from build123d import *

# Parameters (mm, degrees)
SKETCH1_W           = 152.4
SKETCH1_H           = 152.4
BOSS_EXTRUDE1_DEPTH = 101.6
SHELL1_T            = -12.7
SKETCH2_R           = 5.08
CUT_EXTRUDE1_DEPTH  = 189.799073091


with BuildPart() as part:
    # Sketch1 → Boss-Extrude1 (new body)
    with BuildSketch(Plane(origin=(0, 0, 0), x_dir=(1, 0, 0), z_dir=(0, 1, 0))):
        Rectangle(SKETCH1_W, SKETCH1_H)
    extrude(amount=BOSS_EXTRUDE1_DEPTH)

    # Shell1
    shell1_openings = [part.faces().sort_by_distance(p)[0] for p in [
        (0, 101.6, 0),
    ]]
    offset(amount=SHELL1_T, openings=shell1_openings, kind=Kind.INTERSECTION)

    # Sketch2 → Cut-Extrude1 (cut, through all)
    with BuildSketch(Plane.XY.offset(-63.5)):
        with Locations(Location((-53.34, 22.86, 0), (0, 0, 180))):
            Circle(SKETCH2_R)
        with Locations(Location((53.34, 22.86, 0), (0, 0, 180))):
            Circle(SKETCH2_R)
    cut_extrude1 = extrude(amount=CUT_EXTRUDE1_DEPTH, mode=Mode.SUBTRACT)

    # Mirror1: Cut-Extrude1 across plane
    add(cut_extrude1.mirror(Plane.XY), mode=Mode.SUBTRACT)


solid = part.part
The listing builds one solid part. Answer for the finished solid, in the listing's coordinates (mm). A direction names the side the tool comes from. Give positions to 0.01 mm unless a question says otherwise; leave off trailing zeros. Write each loop counter-clockwise with the first axis right and the second up, starting at its lowest first coordinate (ties: lowest second). Pieces come first, ordered by that corner, then holes. Notation, with made-up numbers: (88, 14) - (119, 14) arc R17 ccw to (119, 26) - close; hole circle Ø3 at (61, -8.5). An arc over 180 degrees is marked (long way). Use a Markdown table: item, result.
1. Section B-B on y = 22.86 is taken. Write down the section's boundary in (x, z), plus the area to 3 significant figures.
Values follow:
| item | result |
|---|---|
| outline | (-76.2, -76.2) - (-58.42, -76.2) - (-58.42, -63.5) - (-63.5, -63.5) - (-63.5, 63.5) - (-58.42, 63.5) - (-58.42, 76.2) - (-76.2, 76.2) - close; (-48.26, -76.2) - (48.26, -76.2) - (48.26, -63.5) - (-48.26, -63.5) - close; (-48.26, 63.5) - (48.26, 63.5) - (48.26, 76.2) - (-48.26, 76.2) - close; (58.42, -76.2) - (76.2, -76.2) - (76.2, 76.2) - (58.42, 76.2) - (58.42, 63.5) - (63.5, 63.5) - (63.5, -63.5) - (58.42, -63.5) - close |
| area | 6,580 mm² |
2. Section A-A on x = -53.34 is taken. Write down the section's boundary in (y, z).
Values follow:
| item | result |
|---|---|
| outline | (0, -76.2) - (17.78, -76.2) - (17.78, -63.5) - (12.7, -63.5) - (12.7, 63.5) - (17.78, 63.5) - (17.78, 76.2) - (0, 76.2) - close; (27.94, -76.2) - (101.6, -76.2) - (101.6, -63.5) - (27.94, -63.5) - close; (27.94, 63.5) - (101.6, 63.5) - (101.6, 76.2) - (27.94, 76.2) - close |
3. Each of these flat-tipped pins is pushed along its axis until it touches: P1, Ø2, axis at x = -2.5, z = 56, coming from the -Y side; P2, Ø6, axis at x = 7.5, z = 32.5, coming from the +Y side. Where does it stop, or does it pass through?
Values follow:
| item | result |
|---|---|
| P1 | stops at y = 0 |
| P2 | stops at y = 12.7 |
4. Find the intervals of material crossed by probe 1 along X at (y, z) = (22.86, -68.5); probe 2 along X at (y, z) = (87.5, -28), in increasing order. Write a range as from..to.
Values follow:
| item | result |
|---|---|
| probe 1 | x = -76.2..-58.42, -48.26..48.26, 58.42..76.2 |
| probe 2 | x = -76.2..-63.5, 63.5..76.2 |
5. For a pull along Y with two mould halves and no side action, classify faces 3 (the flat face through (63.5, 57, 1)), 4 (the flat face through (-1, 12.7, -1)), 5 (the cylindrical face through (57.084, 19.427, 69.761)) as released by +Y, released by -Y, zero draft, split by the parting line, or undercut.
Values follow:
| item | result |
|---|---|
| face 3 | zero draft |
| face 4 | released by +Y |
| face 5 | undercut |
6. Section D-D on z = -26 is taken. Write down the section's boundary in (x, y).
Values follow:
| item | result |
|---|---|
| outline | (-76.2, 0) - (76.2, 0) - (76.2, 101.6) - (63.5, 101.6) - (63.5, 12.7) - (-63.5, 12.7) - (-63.5, 101.6) - (-76.2, 101.6) - close |
7. Section C-C on y = 39.5 is taken. Write down the section's boundary in (x, z), plus the area to 3 significant figures.
Values follow:
| item | result |
|---|---|
| outline | (-76.2, -76.2) - (76.2, -76.2) - (76.2, 76.2) - (-76.2, 76.2) - close; hole (-63.5, -63.5) - (63.5, -63.5) - (63.5, 63.5) - (-63.5, 63.5) - close |
| area | 7,100 mm² |
8. A tool of negligible diameter and unlimited length cuts with its end or side. For faces 1 (the flat face through (-1, 57, -63.5)), 2 (the flat face through (-1, 50, 76.2)), from which of +Z, -Z, +X, -X, +Y, -Y can it reach the whole face along a straight path? Write none if from no direction.
Values follow:
| item | result |
|---|---|
| face 1 | +Y |
| face 2 | +Z, +X, -X, +Y, -Y |
